from build123d import *

# Parameters (mm, degrees)
SKETCH_W     = 12.7
SKETCH_H     = 75
SKETCH_R     = 2
PAD_DEPTH    = 12.7
POCKET_DEPTH = 12.701


with BuildPart() as part:
    # Sketch → Pad (new body)
    with BuildSketch(Plane.XY):
        with Locations((6.35, 37.5)):
            Rectangle(SKETCH_W, SKETCH_H)
        with Locations((6.35, 69.5)):
            Circle(SKETCH_R, mode=Mode.SUBTRACT)
        with Locations((6.35, 59.5)):
            Circle(SKETCH_R, mode=Mode.SUBTRACT)
        with Locations((6.35, 15.5)):
            Circle(SKETCH_R, mode=Mode.SUBTRACT)
        with Locations((6.35, 5.5)):
            Circle(SKETCH_R, mode=Mode.SUBTRACT)
    extrude(amount=PAD_DEPTH)

    # Sketch001 (on Face2 of Pad) → Pocket (cut, through all)
    with BuildSketch(Plane.YZ.offset(12.7)):
        with BuildLine():
            ThreePointArc((37.5, 2.85), (45.949747, 6.35), (37.5, 9.85))
            ThreePointArc((37.5, 9.85), (29.050253, 6.35), (37.5, 2.85))
        make_face()
    extrude(amount=-POCKET_DEPTH, mode=Mode.SUBTRACT)


solid = part.part
Build history of the part. All positions in model axes, mm. Give positions to 0.01 mm unless a question says otherwise; leave off trailing zeros. Order: outer loops, then holes, each group sorted by start corner. A loop starts at its lowest first (then second) coordinate and runs counter-clockwise, first axis right, second up. Notation, with made-up numbers: M 45,-8 L 64,-8 A21 cw 64,31 Z; hole C 58.5,62 d4. An arc over 180 degrees is marked long. Use one line per item in the form item = value.
1) Saw through at B-B (x = 6.35). Give the cut face in (y, z).
Calculated:
outline = M 0,0 L 3.5,0 L 3.5,12.7 L 0,12.7 Z; M 7.5,0 L 13.5,0 L 13.5,12.7 L 7.5,12.7 Z; M 17.5,0 L 57.5,0 L 57.5,12.7 L 17.5,12.7 Z; M 61.5,0 L 67.5,0 L 67.5,12.7 L 61.5,12.7 Z; M 71.5,0 L 75,0 L 75,12.7 L 71.5,12.7 Z; hole M 37.5,2.85 A4.95 ccw long 37.5,9.85 A4.95 ccw long Z
2) Probe probe 1 along Z at (x, y) = (8.5, 41); probe 2 along Y at (x, z) = (8, 5); probe 3 along Y at (x, z) = (3, 10.25). List the from-to ranges inside material, lowest first.
Calculated:
probe_1 = 0 to 1.4, 11.3 to 12.7
probe_2 = 0 to 4.37, 6.63 to 14.37, 16.63 to 29.24, 45.76 to 58.37, 60.63 to 68.37, 70.63 to 75
probe_3 = 0 to 30.95, 37.05 to 37.95, 44.05 to 75
3) Saw through at D-D (x = 1.5). Give the cut face in (y, z), plus the area to 3 significant figures.
Calculated:
outline = M 0,0 L 75,0 L 75,12.7 L 0,12.7 Z; hole M 37.5,2.85 A4.95 ccw long 37.5,9.85 A4.95 ccw long Z
area = 813 mm2
4) Saw through at C-C (y = 59.5). Give the cut face in (x, z), plus the area to 3 significant figures.
Calculated:
outline = M 0,0 L 4.35,0 L 4.35,12.7 L 0,12.7 Z; M 8.35,0 L 12.7,0 L 12.7,12.7 L 8.35,12.7 Z
area = 110 mm2
5) Saw through at A-A (z = 6.35). Give the cut face in (x, y), plus the area to 3 significant figures.
Calculated:
outline = M 0,0 L 12.7,0 L 12.7,29.05 L 0,29.05 Z; M 0,45.95 L 12.7,45.95 L 12.7,75 L 0,75 Z; hole C 6.35,5.5 d4; hole C 6.35,15.5 d4; hole C 6.35,59.5 d4; hole C 6.35,69.5 d4
area = 688 mm2
6) Two-plate mould, pull along Y, no slides. Class faces 1 (the face through (6.09, 61.483, 6.261)), 2 (the face through (6, 75, 6)), 3 (the face through (6, 38, 0)): released by +Y, released by -Y, zero draft, split by the parting line, or undercut.
Calculated:
face_1 = undercut
face_2 = released by +Y
face_3 = zero draft
